Input: part model. Units: mm. Frame: model coordinates. Round coordinates to 2 decimals unless told otherwise and drop trailing zeros. Loops run counter-clockwise (first coordinate to the right, second up) from the corner with the lowest first, then second, coordinate; pieces in that order, holes last. Notation, with made-up numbers: (81.5, 57.25) - (124.5, 57.25) arc R23 ccw to (124.5, 75.25) - close; hole circle Ø5 at (22.25, -23.5). An arc over 180 degrees is marked (long way). Write each question's results on one line, items separated by ' | '.
from build123d import *

# Parameters (mm, degrees)
IZIM1_W                     = 100
IZIM1_H                     = 56
IZIM1_R                     = 2.883504547
Y_KSEKLIK_EKSTR_ZYON1_DEPTH = 8
IZIM2_R                     = 11
IZIM2_R_2                   = 1.25
KES_EKSTR_ZYON1_DEPTH       = 10
IZIM3_R                     = 2.6
KES_EKSTR_ZYON2_DEPTH       = 10


with BuildPart() as part:
    # Çizim1 → Yükseklik-Ekstrüzyon1 (new body)
    with BuildSketch(Plane.XY):
        with Locations((7.377917159, -1.029772329)):
            Rectangle(IZIM1_W, IZIM1_H)
        with Locations((7.377917159, 1.970227671)):
            Circle(IZIM1_R, mode=Mode.SUBTRACT)
    extrude(amount=Y_KSEKLIK_EKSTR_ZYON1_DEPTH)

    # Çizim2 → Kes-Ekstrüzyon1 (cut)
    with BuildSketch(Plane(origin=(0, 0, 0), x_dir=(-1, 0, 0), z_dir=(0, 0, -1))):
        with Locations((-7.377917159, 1.970227671)):
            Circle(IZIM2_R)
        with Locations((8.122082841, 17.470227671)):
            Circle(IZIM2_R_2)
        with Locations((7.553397723, -13.529772329)):
            Circle(IZIM2_R_2)
        with Locations((-23.446602277, -12.670089489)):
            Circle(IZIM2_R_2)
        with Locations((-22.877917159, 18.329910511)):
            Circle(IZIM2_R_2)
    extrude(amount=-KES_EKSTR_ZYON1_DEPTH, mode=Mode.SUBTRACT)

    # Çizim3 → Kes-Ekstrüzyon2 (cut)
    with BuildSketch(Plane.XY.offset(8)):
        with Locations((-32.622082841, 19.470227671)):
            Circle(IZIM3_R)
        with Locations((47.377917159, 19.470227671)):
            Circle(IZIM3_R)
        with Locations((47.377917159, -13.529772329)):
            Circle(IZIM3_R)
        with Locations((-32.622082841, -13.529772329)):
            Circle(IZIM3_R)
    extrude(amount=-KES_EKSTR_ZYON2_DEPTH, mode=Mode.SUBTRACT)


solid = part.part
1. Line query: line 1 (Y direction, x = 47, z = 5.75); line 2 (X direction, y = 19, z = 3.25); line 3 (X direction, y = -13, z = 3.5). Output: solid intervals per line, ascending. Write a range as [from, to].
Answer:
line 1: [-29.03, -16.1], [-10.96, 16.9], [22.04, 26.97] | line 2: [-42.62, -35.18], [-30.06, 21.82], [23.93, 44.82], [49.94, 57.38] | line 3: [-42.62, -35.17], [-30.08, -8.69], [-6.42, 22.24], [24.65, 44.83], [49.92, 57.38]
2. Contact query for flat-ended pins moving along their axis: pin 1 (3 mm diameter, centred on x = -32.62, y = 19.47, fed in from +Z); pin 2 (4 mm diameter, centred on x = 15, y = 7, fed in from +Z). Output: stop coordinate, or through.
Answer:
pin 1: through | pin 2: z = 8
3. Mould query, pull axis X, two halves, no side actions, for faces 1 (the cylindrical face through (47.04, 22.05, 4.06)), 2 (the flat face through (57.378, -1, 4)), 3 (the flat face through (-42.622, -1, 4)), 4 (the flat face through (-4, -1, 8)). Classes: pulls with the +X half, pulls with the -X half, needs draft (parallel to the pull), parting line crosses it, or undercut.
Answer:
face 1: undercut | face 2: pulls with the +X half | face 3: pulls with the -X half | face 4: needs draft
4. Section query A-A, the plane y = 3.5. Output: boundary loops of the cut face in (x, z), plus the area to 3 significant figures.
Answer:
outline: (-42.62, 0) - (-3.52, 0) - (-3.52, 8) - (-42.62, 8) - close; (18.27, 0) - (57.38, 0) - (57.38, 8) - (18.27, 8) - close | area: 626 mm^2
5. Section query D-D, the plane x = 49. Output: boundary loops of the cut face in (y, z).
Answer:
outline: (-29.03, 0) - (-15.56, 0) - (-15.56, 8) - (-29.03, 8) - close; (-11.5, 0) - (17.44, 0) - (17.44, 8) - (-11.5, 8) - close; (21.5, 0) - (26.97, 0) - (26.97, 8) - (21.5, 8) - close
6. Section query B-B, the plane x = 11. Output: boundary loops of the cut face in (y, z), plus the area to 3 significant figures.
Answer:
outline: (-29.03, 0) - (-8.42, 0) - (-8.42, 8) - (-29.03, 8) - close; (12.36, 0) - (26.97, 0) - (26.97, 8) - (12.36, 8) - close | area: 282 mm^2
7. Section query C-C, the plane z = 6.5. Count the separate pieces of the cut face and the enclosed holes in it, plus the area to 3 significant figures.
Answer:
separate pieces: 1 | enclosed holes: 9 | area: 5,120 mm^2
